```python
from build123d import *

# Parameters (mm, degrees)
SKETCH2_W                = 50
SKETCH2_H                = 80
BOSS_EXTRUDE1_DEPTH      = 3
M4_CLEARANCE_HOLE1_D     = 4.5
M4_CLEARANCE_HOLE1_DEPTH = 3
M4_CLEARANCE_HOLE1_TIP   = 1.351936393
SKETCH5_R                = 6
CUT_EXTRUDE1_DEPTH       = 3
SKETCH6_R                = 3
CUT_EXTRUDE2_DEPTH       = 3
FILLET1_R                = 2
FILLET2_R                = 25
SKETCH7_W                = 3
SKETCH7_H                = 18
SKETCH7_H_2              = 12
CUT_EXTRUDE3_DEPTH       = 3
M3_CLEARANCE_HOLE1_D     = 3.4
M3_CLEARANCE_HOLE1_DEPTH = 3
M3_CLEARANCE_HOLE1_TIP   = 1.021463052
M3_CLEARANCE_HOLE2_D     = 3.4


with BuildPart() as part:
    # Sketch2 → Boss-Extrude1 (new body)
    with BuildSketch(Plane(origin=(0, 0, 0), x_dir=(1, 0, 0), z_dir=(0, 1, 0))):
        with Locations((25, 40)):
            Rectangle(SKETCH2_W, SKETCH2_H)
    extrude(amount=BOSS_EXTRUDE1_DEPTH)

    # M4 Clearance Hole1
    with Locations(Plane(origin=(0, 3, 0), x_dir=(1, 0, 0), z_dir=(0, 1, 0))):
        with Locations((25, 40)):
            Hole(M4_CLEARANCE_HOLE1_D / 2, depth=M4_CLEARANCE_HOLE1_DEPTH)
            with Locations((0, 0, -(M4_CLEARANCE_HOLE1_DEPTH + M4_CLEARANCE_HOLE1_TIP / 2))):  # 118° drill point
                Cone(0, M4_CLEARANCE_HOLE1_D / 2, M4_CLEARANCE_HOLE1_TIP, mode=Mode.SUBTRACT)

    # Sketch5 → Cut-Extrude1 (cut)
    with BuildSketch(Plane(origin=(0, 3, 0), x_dir=(1, 0, 0), z_dir=(0, 1, 0))):
        with Locations(Location((25, 40, 0), (0, 0, 270))):
            Circle(SKETCH5_R)
    extrude(amount=-CUT_EXTRUDE1_DEPTH, mode=Mode.SUBTRACT)

    # Sketch6 → Cut-Extrude2 (cut)
    with BuildSketch(Plane(origin=(0, 3, 0), x_dir=(1, 0, 0), z_dir=(0, 1, 0))):
        with Locations((25, 34)):
            Circle(SKETCH6_R)
    extrude(amount=-CUT_EXTRUDE2_DEPTH, mode=Mode.SUBTRACT)

    # Fillet1
    fillet1_edges = [part.edges().sort_by_distance(p)[0] for p in [
        (22.09526249, 1.5, -34.75),
        (27.90473751, 1.5, -34.75),
    ]]
    fillet(fillet1_edges, radius=FILLET1_R)

    # Fillet2
    fillet2_edges = [part.edges().sort_by_distance(p)[0] for p in [
        (0, 1.5, 0),
        (50, 1.5, 0),
    ]]
    fillet(fillet2_edges, radius=FILLET2_R - 0.0001)  # a hair under: the kernel refuses the full size

    # Sketch7 → Cut-Extrude3 (cut)
    with BuildSketch(Plane(origin=(0, 3, 0), x_dir=(1, 0, 0), z_dir=(0, 1, 0))):
        with Locations((48.5, 71)):
            Rectangle(SKETCH7_W, SKETCH7_H)
        with Locations((1.5, 71)):
            Rectangle(SKETCH7_W, SKETCH7_H)
        with Locations((48.5, 36)):
            Rectangle(SKETCH7_W, SKETCH7_H_2)
        with Locations((1.5, 36)):
            Rectangle(SKETCH7_W, SKETCH7_H_2)
    extrude(amount=-CUT_EXTRUDE3_DEPTH, mode=Mode.SUBTRACT)

    # M3 Clearance Hole1
    with Locations(Plane(origin=(0, 3, 0), x_dir=(1, 0, 0), z_dir=(0, 1, 0))):
        with Locations((25, 48.3), (25, 20.5)):
            Hole(M3_CLEARANCE_HOLE1_D / 2, depth=M3_CLEARANCE_HOLE1_DEPTH)
            with Locations((0, 0, -(M3_CLEARANCE_HOLE1_DEPTH + M3_CLEARANCE_HOLE1_TIP / 2))):  # 118° drill point
                Cone(0, M3_CLEARANCE_HOLE1_D / 2, M3_CLEARANCE_HOLE1_TIP, mode=Mode.SUBTRACT)

    # M3 Clearance Hole2 (through all)
    with Locations(Plane(origin=(0, 3, 0), x_dir=(1, 0, 0), z_dir=(0, 1, 0))):
        with Locations((1.5, 49.5), (48.5, 49.5)):
            Hole(M3_CLEARANCE_HOLE2_D / 2)


solid = part.part
```
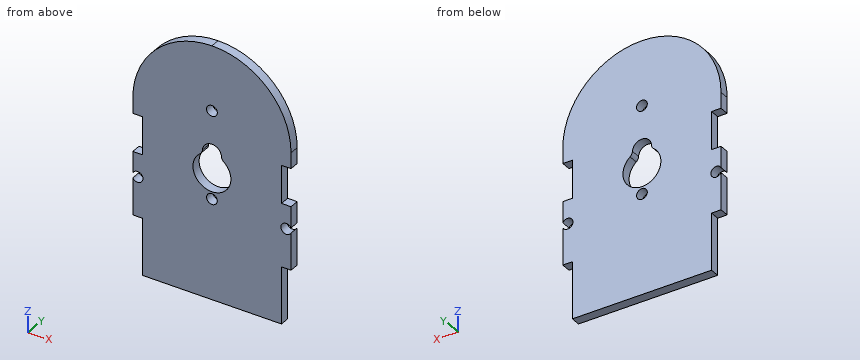
Here's how the part is built. I have some questions about the finished solid (model axes, mm). Round coordinates to 2 decimals unless told otherwise and drop trailing zeros. Loops run counter-clockwise (first coordinate to the right, second up) from the corner with the lowest first, then second, coordinate; pieces in that order, holes last. Notation, with made-up numbers: (30.25, -15.5) -> (46.25, -15.5) arc R29 cw to (46.25, 18.5) -> close; hole circle Ø9 at (12.5, 4). An arc over 180 degrees is marked (long way). Answer as CSV lines item,"result".
1. If we section it at B-B on x = 48.5: Please give me the cut outline in (y, z), plus the area to 3 significant figures.
Final values:
outline,"(0, -62) -> (3, -62) -> (3, -51.2) -> (0, -51.2) -> close; (0, -47.8) -> (3, -47.8) -> (3, -42) -> (0, -42) -> close; (0, -30) -> (3, -30) -> (3, -16.47) -> (0, -16.47) -> close"
area,"90.4 mm^2"
2. If we section it at D-D on y = 0.6: Count the separate pieces of the cut face and the enclosed holes in it, plus the area to 3 significant figures.
Final values:
separate pieces,"1"
enclosed holes,"3"
area,"3,390 mm^2"
3. If we section it at A-A on z = -40: Please give me the cut outline in (x, y).
Final values:
outline,"(3, 0) -> (19, 0) -> (19, 3) -> (3, 3) -> close; (31, 0) -> (47, 0) -> (47, 3) -> (31, 3) -> close"
4. If we section it at C-C on z = -68: Please give me the cut outline in (x, y), plus the area to 3 significant figures.
Final values:
outline,"(3, 0) -> (47, 0) -> (47, 3) -> (3, 3) -> close"
area,"132 mm^2"
5. If I drill on L1, parallel to Z at x = 25, y = 2.2; L2, parallel to X at y = 2.35, z = -40; L3, parallel to Z at x = 30.5, y = 0.7, over which ranges is the centre line in solid material (lowest first)?
Final values:
L1,"z = -80 to -50, -46.6 to -46, -31 to -22.2, -18.8 to 0"
L2,"x = 3 to 19, 31 to 47"
L3,"z = -80 to -42.4, -37.6 to -0.61"
6. For pin 1 (0.9 mm diameter, centred on x = 2, y = 1, fed in from -Z); pin 2 (5.5 mm diameter, centred on x = 48.5, z = -49.5, fed in from -Y); pin 3 (1.5 mm diameter, centred on x = 2, y = 1.5, fed in from +Z), each with a flat end and sliding along its axis, tell me the tip position at first contact or that it passes through.
Final values:
pin 1,"stops at z = -62"
pin 2,"stops at y = 0"
pin 3,"stops at z = -13.6"
